Could you check a few things on this model? Use its own coordinates, in mm. Give positions to 0.01 mm unless a question says otherwise; leave off trailing zeros. Loops run counter-clockwise (first coordinate to the right, second up) from the corner with the lowest first, then second, coordinate; pieces in that order, holes last.
1. Imagine slicing it at C-C (z = 56.5). List the corners of the cut face in (x, y) for me.
2. Imagine slicing it at D-D (x = -5.25). List the corners of the cut face in (y, z) for me (3 decimals), plus the area to 3 significant figures.
3. I need wall thicknesses on line 1 along Y through (x, z) = (-1, 114.3) (3 decimals); line 2 along Z through (x, y) = (-0.5, 0) (3 decimals); line 3 along Z through (x, y) = (7.5, 5). Which ranges of each line are inside material? Lowest first, please.
4. For P1, Ø3, axis at y = 1, z = -9.5, coming from the +X side (3 decimals); P2, Ø5, axis at x = 1, z = -4, coming from the +Y side (3 decimals); P3, Ø1, axis at x = -5, y = 6.5, coming from the -Z side, each with a flat end and sliding along its axis, tell me the tip position at first contact or that it passes through.
5. Imagine slicing it at A-A (x = 0). List the corners of the cut face in (y, z) for me (3 decimals).
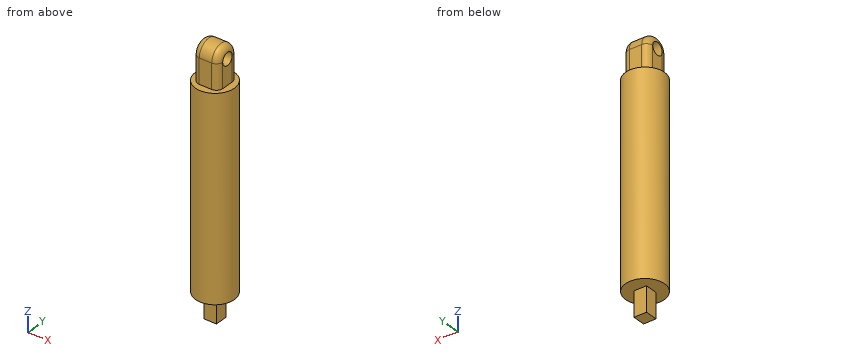
Autodesk Inventor part; units mm, degrees
ref_plane "YZ Plane" through (0, 0, 0) normal (1, 0, 0) x (0, 1, 0)
ref_plane "XZ Plane" through (0, 0, 0) normal (0, 1, 0) x (-1, 0, 0)
ref_plane "XY Plane" through (0, 0, 0) normal (0, 0, 1) x (1, 0, 0)
sketch "Sketch1" plane through (0, 0, 0) normal (0, 0, 1) x (1, 0, 0)
  circle A0 centre (0, 0) radius 6.0688
extrude "Extrusion1" add sketch "Sketch1" along normal blind 101.6
sketch "Sketch2" plane through (0, 0, 101.6) normal (0, 0, 1) x (1, 0, 0)
  line L0 (-6.0688, 6.0688) -> (6.0688, 6.0688)
  line L1 (6.0688, 6.0688) -> (6.0688, -6.0688)
  line L2 (6.0688, -6.0688) -> (-6.0688, -6.0688)
  line L3 (-6.0688, -6.0688) -> (-6.0688, 6.0688)
extrude "Extrusion2" add sketch "Sketch2" along normal blind 12.7
sketch "Sketch3" plane through (6.0688, -6.0688, 101.6) normal (1, 0, 0) x (0, 0, -1)
  line L0 (-12.7, 12.1376) -> (-12.7, 0)
  circle A0 centre (-12.7, 6.0688) radius 3.175
  point P0 (101.6, 6.0688)
  dimension "d4" = 6.35
extrude "Extrusion3" cut sketch "Sketch3" against normal blind 12.7
sketch "Sketch4" plane through (6.0688, -6.0688, 101.6) normal (1, 0, 0) x (0, 0, -1)
  arc A0 (-12.7, 2.8938) -> (-12.7, 9.2438) centre (-12.7, 6.0688) ccw
  circle A1 centre (-12.7, 6.0688) radius 3.175
  circle A2 centre (-12.7, 6.0688) radius 6.0688
  point P0 (101.6, 6.0688)
extrude "Extrusion4" add sketch "Sketch4" against normal blind 12.7
sketch "Sketch5" plane through (-6.0688, 0, 101.6) normal (-1, 0, 0) x (0, 0, 1)
  arc A0 (12.7, 6.0688) -> (12.7, -6.0688) centre (12.7, 0) ccw
  line L0 (0, 6.0688) -> (12.7, 6.0688)
  line L1 (0, 0) -> (0, 6.0688)
  line L2 (0, -6.0688) -> (0, 0)
  line L3 (0, -6.0688) -> (12.7, -6.0688)
  line L4 (0, 6.0688) -> (38.3978, 6.0688)
  line L5 (38.3978, 6.0688) -> (38.3978, -6.0688)
  line L6 (38.3978, -6.0688) -> (0, -6.0688)
  line L7 (0, -6.0688) -> (0, 6.0688)
  point P0 (-101.6, 0)
extrude "Extrusion5" cut sketch "Sketch5" along normal blind 12.7 contours L4 L5 L6 A0
sketch "Sketch6" plane through (0, 0, 0) normal (0, 0, -1) x (-1, 0, 0)
  circle A0 centre (0, 0) radius 6.0688
  line L0 (0, 0) -> (0, 3.175)
  line L1 (0, 3.175) -> (-3.175, 3.175)
  line L2 (-3.175, 3.175) -> (3.175, 3.175)
  line L3 (3.175, 3.175) -> (3.175, -3.175)
  line L4 (3.175, -3.175) -> (-3.175, -3.175)
  line L5 (-3.175, -3.175) -> (-3.175, 3.175)
  dimension "d11" = 3.175
  dimension "d12" = 3.175
  dimension "d13" = 6.35
  dimension "d14" = 6.35
extrude "Extrusion6" add sketch "Sketch6" along normal blind 12.7 contours L2 L3 L4 L5 L1
fillet "Fillet1" radius 3.175 6 edges at (6.0688, 6.0688, 107.95) (6.0688, 0, 120.3688) (6.0688, -6.0688, 107.95) (-6.0688, 6.0688, 107.95) (-6.0688, 0, 120.3688) (-6.0688, -6.0688, 107.95)
sketch "Sketch7" plane through (0, 0, 0) normal (0, 0, -1) x (-1, 0, 0)
  circle A0 centre (0, 0) radius 6.0688
  circle A1 centre (0, 0) radius 9.906
  dimension "d18" = 19.812
extrude "Extrusion7" add sketch "Sketch7" against normal blind 101.6
sketch "Sketch8" plane through (0, 0, 101.6) normal (0, 0, 1) x (1, 0, 0)
  circle A0 centre (0, 0) radius 9.906
extrude "Extrusion8" cut sketch "Sketch8" along normal blind 101.6
sketch "Sketch9" plane through (0, 0, 101.6) normal (0, 0, 1) x (1, 0, 0)
  circle A0 centre (0, 0) radius 9.906
  circle A1 centre (0, 0) radius 6.35
  line L0 (-6.35, 6.35) -> (6.35, 6.35)
  line L1 (6.35, 6.35) -> (6.35, -6.35)
  line L2 (6.35, -6.35) -> (-6.35, -6.35)
  line L3 (-6.35, -6.35) -> (-6.35, 6.35)
  dimension "d23" = 12.7
extrude "Extrusion9" add sketch "Sketch9" along normal blind 12.7 contours A1 | L1 L2 A1 | A1 L0 L1 | A1 L3 L0 | L2 L3 A1
sketch "Sketch10" plane through (6.35, -6.35, 101.6) normal (1, 0, 0) x (0, 0, -1)
  line L0 (-12.7, 12.7) -> (-12.7, 0)
  circle A0 centre (-12.7, 6.35) radius 3.175
  point P0 (101.6, 6.35)
  dimension "d26" = 6.35
extrude "Extrusion10" cut sketch "Sketch10" against normal blind 12.7
sketch "Sketch11" plane through (6.35, -6.35, 101.6) normal (1, 0, 0) x (0, 0, -1)
  arc A0 (-12.7, 3.175) -> (-12.7, 9.525) centre (-12.7, 6.35) ccw
  circle A1 centre (-12.7, 6.35) radius 3.175
  circle A2 centre (-12.7, 6.35) radius 6.35
  point P0 (101.6, 6.35)
extrude "Extrusion11" add sketch "Sketch11" against normal blind 12.7
fillet "Fillet2" radius 3.175 6 edges at (6.35, 6.35, 107.95) (6.35, 0, 120.65) (6.35, -6.35, 107.95) (-6.35, 6.35, 107.95) (-6.35, 0, 120.65) (-6.35, -6.35, 107.95)
properties part number "linac arm1"
Derived:
1. outline: circle Ø19.81 at (0, 0)
2. outline: (-8.4, 0) - (8.4, 0) - (8.4, 101.6) - (5.578, 101.6) - (5.578, 114.3) arc R5.578 ccw to (-5.578, 114.3) - (-5.578, 101.6) - (-8.4, 101.6) - close; hole circle Ø6.35 at (0, 114.3)
2. area: 1,870 mm2
3. line 1: y = -6.35 to -3.175, 3.175 to 6.35
3. line 2: z = -12.7 to 111.125, 117.475 to 120.65
3. line 3: z = 0 to 101.6
4. P1: stops at x = 3.175
4. P2: stops at y = 3.175
4. P3: stops at z = 0
5. outline: (-9.906, 0) - (-3.175, 0) - (-3.175, -12.7) - (3.175, -12.7) - (3.175, 0) - (9.906, 0) - (9.906, 101.6) - (6.35, 101.6) - (6.35, 114.3) arc R6.35 ccw to (-6.35, 114.3) - (-6.35, 101.6) - (-9.906, 101.6) - close; hole circle Ø6.35 at (0, 114.3)
